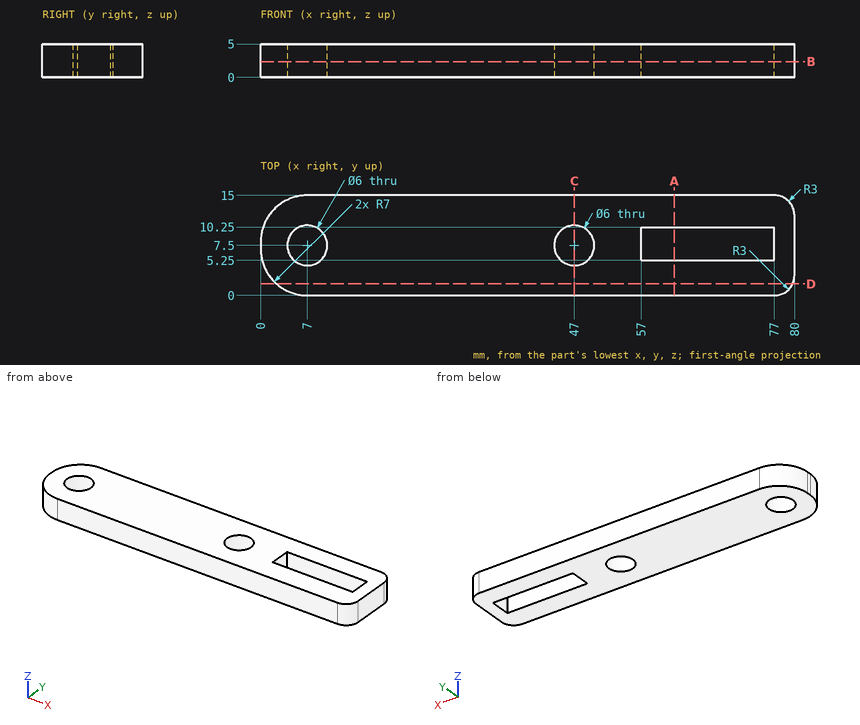
Answer from the drawing. Dimensions are ordinates in mm from the lowest x, y and z of the part. Give positions to 0.01 mm unless a question says otherwise; leave off trailing zeros. Loops run counter-clockwise (first coordinate to the right, second up) from the corner with the lowest first, then second, coordinate; pieces in that order, holes last. Notation, with made-up numbers: (4, 10.5) -> (61, 10.5) arc R17 ccw to (61, 27.5) -> close; hole circle Ø3 at (-29, 70.25). An arc over 180 degrees is marked (long way). Answer as CSV lines item,"result".
Item 1: Find section D-D on y = 1.75. Give the vertices of the cut face in (x, z).
Returned:
outline,"(2.37, 0) -> (79.73, 0) -> (79.73, 5) -> (2.37, 5) -> close"
Item 2: Consider line 1 (Y direction, x = 47, z = 3.85); line 2 (X direction, y = 6.75, z = 0.2); line 3 (X direction, y = 9, z = 1.3). Determine where each line is inside the solid, lowest interval first. Write a range as [from, to].
Returned:
line 1,"y = [0, 4.5], [10.5, 15]"
line 2,"x = [0, 4.1], [9.9, 44.1], [49.9, 57], [77, 80]"
line 3,"x = [0.07, 4.4], [9.6, 44.4], [49.6, 57], [77, 80]"
Item 3: Each of these flat-tipped pins is pushed along its axis until it touches: pin 1 (3.5 mm diameter, centred on x = 7, y = 7.5, fed in from +Z); pin 2 (1.5 mm diameter, centred on y = 4, z = 1.5, fed in from -X). Where does it stop, or does it pass through?
Returned:
pin 1,"passes through"
pin 2,"stops at x = 0.37"
Item 4: Find section A-A on x = 62. Give the vertices of the cut face in (y, z), plus the area to 3 significant figures.
Returned:
outline,"(0, 0) -> (5.25, 0) -> (5.25, 5) -> (0, 5) -> close; (10.25, 0) -> (15, 0) -> (15, 5) -> (10.25, 5) -> close"
area,"50.0 mm²"
Item 5: Find section B-B on z = 2.35. Give the vertices of the cut face in (x, y).
Returned:
outline,"(0, 7) arc R7 ccw to (7, 0) -> (77, 0) arc R3 ccw to (80, 3) -> (80, 12) arc R3 ccw to (77, 15) -> (7, 15) arc R7 ccw to (0, 8) -> close; hole circle Ø6 at (7, 7.5); hole circle Ø6 at (47, 7.5); hole (57, 5.25) -> (77, 5.25) -> (77, 10.25) -> (57, 10.25) -> close"
Item 6: Find section C-C on x = 47. Give the vertices of the cut face in (y, z).
Returned:
outline,"(0, 0) -> (4.5, 0) -> (4.5, 5) -> (0, 5) -> close; (10.5, 0) -> (15, 0) -> (15, 5) -> (10.5, 5) -> close"
